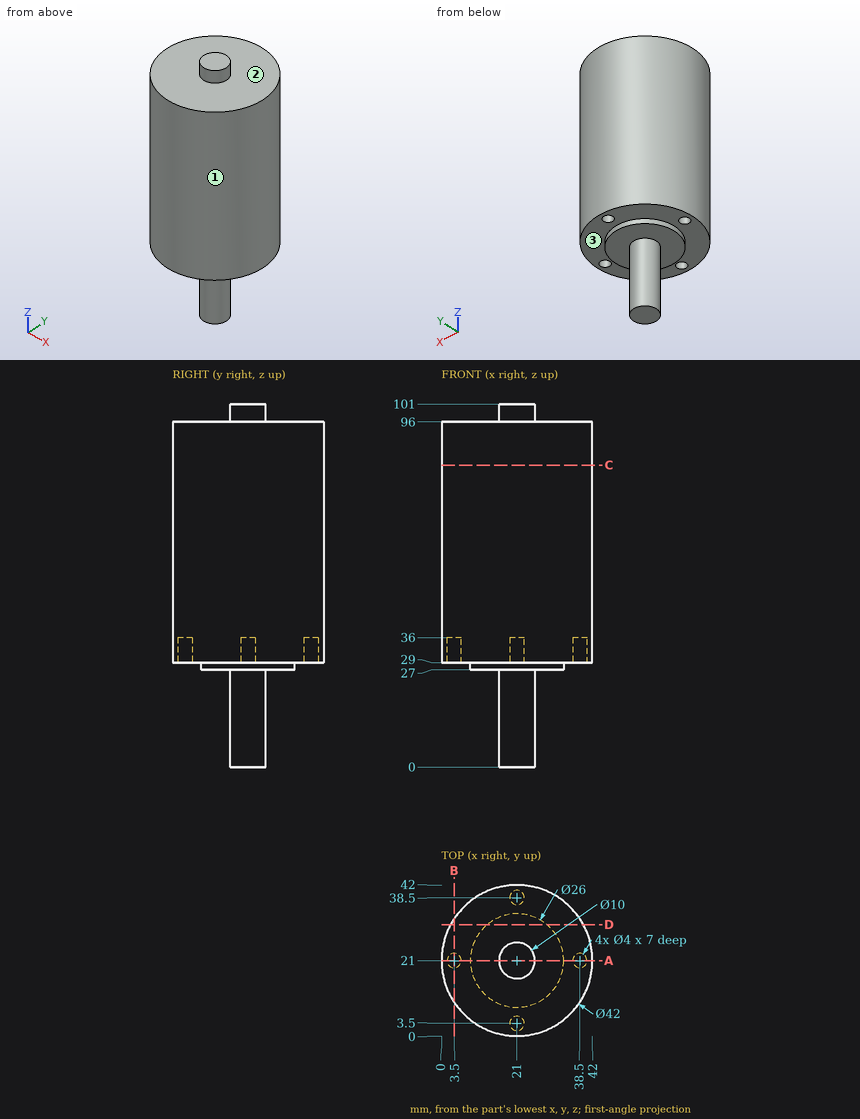
Geometry: see drawing. Coordinates: mm, zero at the bounding-box minimum. A direction names the side the tool comes from. Give positions to 0.01 mm unless a question says otherwise; leave off trailing zeros. Loops run counter-clockwise (first coordinate to the right, second up) from the corner with the lowest first, then second, coordinate; pieces in that order, holes last. Notation, with made-up numbers: (11, 29.25) - (68, 29.25) arc R26 ccw to (68, 44.25) - close; hole circle Ø1 at (-6, -13). An arc over 180 degrees is marked (long way). One line per question, with ' | ' between items. Start each with the question number.
(1) Contact query for flat-ended pins moving along their axis: pin 1 (6 mm diameter, centred on x = 8.5, z = 73.5, fed in from -Y); pin 2 (3 mm diameter, centred on x = 20, y = 2.5, fed in from -Z); pin 3 (5 mm diameter, centred on x = 19, z = 88, fed in from +Y). Output: stop coordinate, or through.
(2) Section query D-D on y = 31. Return loops of the section in (x, z).
(3) Section query A-A on y = 21. Return loops of the section in (x, z), then the cut area to 3 significant figures.
(4) Ray query, line 1 (Y direction, x = 21, z = 33.5); line 2 (Z direction, x = 9.5, y = 10.5); line 3 (Y direction, x = 38, z = 34). Return the intervals inside material, ascending. Write a range as from..to.
(5) Section query C-C on z = 84. Return loops of the section in (x, y).
(6) Section query B-B on x = 3.5. Return loops of the section in (y, z).
(7) Reachability of the marked faces 1, 2 and 3 from +Z, -Z, +X, -X, +Y, -Y: full face, straight path, thin tool, end or side. Return the list, or none.
The answers:
1) pin 1: y = 2.27 | pin 2: z = 29 | pin 3: y = 42
2) outline: (2.53, 29) - (12.69, 29) - (12.69, 27) - (29.31, 27) - (29.31, 29) - (39.47, 29) - (39.47, 96) - (2.53, 96) - close
3) outline: (0, 29) - (1.5, 29) - (1.5, 36) - (5.5, 36) - (5.5, 29) - (8, 29) - (8, 27) - (16, 27) - (16, 0) - (26, 0) - (26, 27) - (34, 27) - (34, 29) - (36.5, 29) - (36.5, 36) - (40.5, 36) - (40.5, 29) - (42, 29) - (42, 96) - (26, 96) - (26, 101) - (16, 101) - (16, 96) - (0, 96) - close | area: 3,130 mm2
4) line 1: 0..1.5, 5.5..36.5, 40.5..42 | line 2: 29..96 | line 3: 8.67..19.06, 22.94..33.33
5) outline: circle Ø42 at (21, 21)
6) outline: (9.39, 29) - (19, 29) - (19, 36) - (23, 36) - (23, 29) - (32.61, 29) - (32.61, 96) - (9.39, 96) - close
7) face 1: +Z, -Z | face 2: +Z | face 3: -Z
